from build123d import *

# Parameters (mm, degrees)
F0_R     = 38.1
F0_R_2   = 1.27
F1_DEPTH = 6.35


with BuildPart() as f1:
    # F0 (on Top) → F1 (new body)
    with BuildSketch(Plane.XY):
        with Locations((-6.822567, 15.864339)):
            Circle(F0_R)
        with BuildLine():
            ThreePointArc((-11.720609, 10.02708), (-9.428761, 8.703881), (-6.822567, 8.244339))
            Line((-6.822567, 8.244339), (-6.822567, -17.155661))
            ThreePointArc((-6.822567, -17.155661), (-18.116073, -15.164312), (-28.047414, -9.430449))
            Line((-28.047414, -9.430449), (-11.720609, 10.02708))
        make_face(mode=Mode.SUBTRACT)
        with BuildLine():
            ThreePointArc((-14.326803, 17.187538), (-14.326803, 14.54114), (-13.421681, 12.054339))
            Line((-13.421681, 12.054339), (-35.418726, -0.645661))
            ThreePointArc((-35.418726, -0.645661), (-39.340919, 10.130476), (-39.340919, 21.598202))
            Line((-39.340919, 21.598202), (-14.326803, 17.187538))
        make_face(mode=Mode.SUBTRACT)
        with BuildLine():
            ThreePointArc((-4.216374, 8.703881), (-1.924526, 10.02708), (-0.223454, 12.054339))
            Line((-0.223454, 12.054339), (21.773591, -0.645661))
            ThreePointArc((21.773591, -0.645661), (14.402279, -9.430449), (4.470938, -15.164312))
            Line((4.470938, -15.164312), (-4.216374, 8.703881))
        make_face(mode=Mode.SUBTRACT)
        with BuildLine():
            ThreePointArc((-9.428761, 23.024796), (-11.720609, 21.701597), (-13.421681, 19.674339))
            Line((-13.421681, 19.674339), (-35.418726, 32.374339))
            ThreePointArc((-35.418726, 32.374339), (-28.047414, 41.159126), (-18.116073, 46.892989))
            Line((-18.116073, 46.892989), (-9.428761, 23.024796))
        make_face(mode=Mode.SUBTRACT)
        with Locations((-6.822567, 15.864339)):
            Circle(F0_R_2, mode=Mode.SUBTRACT)
        with BuildLine():
            ThreePointArc((0.681668, 14.54114), (0.681668, 17.187538), (-0.223454, 19.674339))
            Line((-0.223454, 19.674339), (21.773591, 32.374339))
            ThreePointArc((21.773591, 32.374339), (25.695785, 21.598202), (25.695785, 10.130476))
            Line((25.695785, 10.130476), (0.681668, 14.54114))
        make_face(mode=Mode.SUBTRACT)
        with BuildLine():
            ThreePointArc((-6.822567, 48.884339), (4.470938, 46.892989), (14.402279, 41.159126))
            Line((14.402279, 41.159126), (-1.924526, 21.701597))
            ThreePointArc((-1.924526, 21.701597), (-4.216374, 23.024796), (-6.822567, 23.484339))
            Line((-6.822567, 23.484339), (-6.822567, 48.884339))
        make_face(mode=Mode.SUBTRACT)
    extrude(amount=F1_DEPTH)


solid = f1.part
Here's how the part is built. I have some questions about the finished solid (model axes, mm). A direction names the side the tool comes from. Coordinates: 2 decimals unless noted, no trailing zeros. Write each loop counter-clockwise with the first axis right and the second up, starting at its lowest first coordinate (ties: lowest second). Pieces come first, ordered by that corner, then holes.
Item 1: On a 3-axis mill with a long thin cutter (end or side, diameter ignored), from which of +Z, -Z, +X, -X, +Y, -Y can I reach the whole of each face in a straight line? I mean faces 4 (the flat face through (-7, 25, 0)), 5 (the cylindrical face through (14.526, -9.326, 3.131)). Say none if no direction works.
Item 2: I want a section at A-A on y = -4. Write out the boundary of the cut face in (x, z).
Item 3: I want a section at D-D on z = 2. Write out the boundary of the cut face in (x, y), and give its area (3 significant figures).
Item 4: I want a section at C-C on y = 5. Write out the boundary of the cut face in (x, z).
Item 5: If I drill on line 1 (Y direction, x = -7, z = 1); line 2 (X direction, y = -7, z = 4.5); line 3 (X direction, y = 44.5, z = 3), over which ranges is the centre line in solid material (lowest first)?
Item 6: I want a section at B-B on x = 13. Write out the boundary of the cut face in (y, z), and give its area (3 significant figures).
Item 7: Will these pins go through, and if not, where does the flat tip stop? pin 1 (2 mm diameter, centred on y = -4, z = 1.5, fed in from -X); pin 2 (2 mm diameter, centred on x = -0.5, z = 5.5, fed in from -Y); pin 3 (3 mm diameter, centred on y = 11.5, z = 5.5, fed in from -X).
Item 8: If we mould it in two halves opening along X, with no side actions, what happens to faces 1 (the flat face through (-7, 25, 6.35)), 2 (the flat face through (13.4, 12.3, 3.1)), 3 (the cylindrical face through (-15.08, -21.33, 3.13))? For each: +X half, -X half, draft (parallel to the pull), parting line (faces both ways), or undercut.
Findings below:
1. face 4: -Z, +X, -X, +Y, -Y
1. face 5: +Z, -Z
2. outline: (-39.33, 0) - (-23.49, 0) - (-23.49, 6.35) - (-39.33, 6.35) - close; (-6.82, 0) - (0.41, 0) - (0.41, 6.35) - (-6.82, 6.35) - close; (19.55, 0) - (25.69, 0) - (25.69, 6.35) - (19.55, 6.35) - close
3. outline: circle Ø76.2 at (-6.82, 15.86); hole (-39.34, 21.6) arc R33.02 ccw to (-35.42, -0.65) - (-13.42, 12.05) arc R7.62 cw to (-14.33, 17.19) - close; hole (-35.42, 32.37) - (-13.42, 19.67) arc R7.62 cw to (-9.43, 23.02) - (-18.12, 46.89) arc R33.02 ccw to start; hole (-28.05, -9.43) arc R33.02 ccw to (-6.82, -17.16) - (-6.82, 8.24) arc R7.62 cw to (-11.72, 10.03) - close; hole circle Ø2.54 at (-6.82, 15.86); hole (-6.82, 23.48) arc R7.62 cw to (-1.92, 21.7) - (14.4, 41.16) arc R33.02 ccw to (-6.82, 48.88) - close; hole (-4.22, 8.7) - (4.47, -15.16) arc R33.02 ccw to (21.77, -0.65) - (-0.22, 12.05) arc R7.62 cw to start; hole (-0.22, 19.67) arc R7.62 cw to (0.68, 14.54) - (25.7, 10.13) arc R33.02 ccw to (21.77, 32.37) - close
3. area: 2,390 mm2
4. outline: (-43.34, 0) - (-38, 0) - (-38, 6.35) - (-43.34, 6.35) - close; (-25.64, 0) - (-15.94, 0) - (-15.94, 6.35) - (-25.64, 6.35) - close; (-6.82, 0) - (-2.87, 0) - (-2.87, 6.35) - (-6.82, 6.35) - close; (12, 0) - (29.7, 0) - (29.7, 6.35) - (12, 6.35) - close
5. line 1: y = -22.24 to -17.16, 8.25 to 14.61, 17.12 to 53.96
5. line 2: x = -37.3 to -26.01, -6.82 to 1.5, 17 to 23.65
5. line 3: x = -31.95 to -23.26, -17.25 to -6.82, 9.62 to 18.31
6. outline: (-16.67, 0) - (-10.54, 0) - (-10.54, 6.35) - (-16.67, 6.35) - close; (4.42, 0) - (12.37, 0) - (12.37, 6.35) - (4.42, 6.35) - close; (27.31, 0) - (39.49, 0) - (39.49, 6.35) - (27.31, 6.35) - close; (42.27, 0) - (48.4, 0) - (48.4, 6.35) - (42.27, 6.35) - close
6. area: 206 mm2
7. pin 1: stops at x = -39.92
7. pin 2: stops at y = -21.86
7. pin 3: stops at x = -44.81
8. face 1: draft
8. face 2: undercut
8. face 3: parting line
